```python
from build123d import *

# Parameters (mm, degrees)
BASEHEAD_DEPTH = 17.78


with BuildPart() as part:
    # Sketch1 → BaseHead (new body)
    with BuildSketch(Plane(origin=(0, 0, 0), x_dir=(0, 0, -1), z_dir=(1, 0, 0))):
        Polygon((19.05, 10.998522628), (19.05, -10.998522628), (0, -21.997045256), (-19.05, -10.998522628), (-19.05, 10.998522628), (0, 21.997045256), align=None)
    extrude(amount=BASEHEAD_DEPTH)

    # BodySke → BaseBody (revolve)
    with BuildSketch(Plane.XY):
        Polygon((0, 0), (93.98, 0), (93.98, 10.8077), (92.0877, 12.7), (0, 12.7), align=None)
    revolve(axis=Axis((0, 0, 0), (1, 0, 0)))

    # Sketch3 → HeadChamfer (revolve, cut)
    with BuildSketch(Plane.XY):
        Polygon((0, 19.05), (5.367651581, 28.347045256), (5.367651581, 34.697045256), (-12.7, 34.697045256), (-12.7, 19.05), align=None)
    revolve(axis=Axis((0, 0, 0), (1, 0, 0)), mode=Mode.SUBTRACT)


solid = part.part
```
Source: CAD feature listing. Evaluate the final solid. Frame: model axes, mm. A direction names the side the tool comes from. Give positions to 0.01 mm unless a question says otherwise; leave off trailing zeros. Order: outer loops, then holes, each group sorted by start corner. A loop starts at its lowest first (then second) coordinate and runs counter-clockwise, first axis right, second up. Notation, with made-up numbers: (-26.75, 13.25) -> (-0.75, 13.25) arc R31 cw to (-0.75, 50.25) -> close; hole circle Ø6 at (-36.75, -8.75). An arc over 180 degrees is marked (long way). Use a Markdown table: item, result.
Q1. Access query for faces 1 (the face through (0.41, -9.84, 17.14)), 2 (the face through (17.78, -9.5, -8.7)). Directions: +Z, -Z, +X, -X, +Y, -Y. A direction counts if a zero-diameter tool reaches every point of the face in a straight line with its end or side. Return the directions, or none.
A:
| item | result |
|---|---|
| face 1 | +Z, -X, -Y |
| face 2 | +X |
Q2. First-contact query: P1, Ø10, axis at x = 67.5, y = -1.5, coming from the -Z side; P2, Ø5, axis at x = 11, z = 4, coming from the +Y side; P3, Ø5, axis at x = 14, y = -11.5, coming from the +Z side; P4, Ø4, axis at x = 40, z = -5.5, coming from the +Y side. Flat tips, straight axial feed; report the tip coordinate or a pass-through.
A:
| item | result |
|---|---|
| P1 | z = -12.7 |
| P2 | y = 21.13 |
| P3 | z = 19.05 |
| P4 | y = 12.21 |
Q3. Section A-A (x = 61.5). Return the cut outline in (y, z).
A:
| item | result |
|---|---|
| outline | circle Ø25.4 at (0, 0) |
Q4. Material intervals for line 1 (X direction, y = -11.5, z = 9.5); line 2 (X direction, y = -1.5, z = 11.5); line 3 (Z direction, x = 78, y = 1), sorted ascending. Write a range as [from, to].
A:
| item | result |
|---|---|
| line 1 | [0, 17.78] |
| line 2 | [0, 93.19] |
| line 3 | [-12.66, 12.66] |
